Autodesk Inventor part; units mm, degrees
ref_plane "Work Plane1" through (0, 0, 10) normal (0, 0, 1) x (1, 0, 0)
ref_plane "YZ Plane" through (0, 0, 0) normal (1, 0, 0) x (0, 1, 0)
ref_plane "XZ Plane" through (0, 0, 0) normal (0, 1, 0) x (-1, 0, 0)
ref_plane "Work Plane1" through (0, 0, 10) normal (0, 0, 1) x (1, 0, 0)
sketch "Sketch2" plane through (0, 0, 10) normal (0, 0, 1) x (1, 0, 0)
  line L0 (0, 0) -> (30, 0)
  line L1 (30, 0) -> (30, 3)
  line L2 (30, 3) -> (0, 3)
  line L3 (0, 3) -> (0, 0)
  line L4 (30, 13) -> (0, 13)
  dimension "d11" = 30
  dimension "d12" = 3
  dimension "d13" = 10
revolve "Revolution1" add sketch "Sketch2" angle 360 about axis through (30, 13, 10) along (-1, 0, 0)
sketch "Sketch3" plane through (0, 0, 10) normal (0, 0, 1) x (1, 0, 0)
  line L0 (18.6699, 0) -> (35.6699, 0)
  line L1 (35.6699, 0) -> (35.6699, 5)
  line L2 (35.6699, 5) -> (18.6699, 5)
  line L3 (18.6699, 5) -> (28, 2.5)
  line L4 (28, 2.5) -> (18.6699, 0)
  line L5 (0, 26) -> (0, 0)
  line L6 (-3.0148, 0) -> (-5.3111, 0)
  dimension "d17" = 17
  dimension "d19" = 15
  dimension "d20" = 15
  dimension "d21" = 2.5
  dimension "d23" = 28
  dimension "d24" = 5
  dimension "d25" = 5.3111
  dimension "d26" = 7.6699
extrude "Extrusion2" cut sketch "Sketch3" along normal mid plane 13
equation "\"d20\" = d19"
properties part number "Whistle 1.3"
Build history of the part. All positions in model axes, mm. A direction names the side the tool comes from. Round coordinates to 2 decimals unless told otherwise and drop trailing zeros. Loops run counter-clockwise (first coordinate to the right, second up) from the corner with the lowest first, then second, coordinate; pieces in that order, holes last. Notation, with made-up numbers: (9.5, 83.5) -> (67.5, 83.5) arc R21 ccw to (67.5, 102.5) -> close; hole circle Ø4 at (81.25, 16). An arc over 180 degrees is marked (long way). Use CSV: the item, a comma, the result in double quotes. Start each with the question number.
Q1. Mould opens along Y. For faces 4 (the face through (30, 23, 12)), 5 (the face through (15.21, 25.987, 9.428)), 6 (the face through (26.38, 2.934, 9.909)), 7 (the face through (15, 23, 10)) say: +Y half, -Y half, draft (parallel to the pull), parting line (faces both ways), or undercut.
Q2. Flat gauge pins, fed straight in: pin 1 Ø2 at (x, z) = (13, 0) entering from -Y; pin 2 Ø5 at (x, z) = (21.5, 4.5) entering from -Y; pin 3 Ø3.5 at (x, y) = (23.5, 3.5) entering from +Z. Where does each tip first touch, or does it go through?
Q3. Which spindle directions (+Z, -Z, +X, -X, +Y, -Y) get a long thin tool onto all of the face, cutting with end or side? Do faces 1 (the face through (27, 4, 16.5)), 2 (the face through (24.437, 1.545, 9.909)), 3 (the face through (0, 6, 2)). Say none if no direction does.
Q4. Saw through at C-C on x = 19.5. Give the cut face in (y, z), and give its area (3 significant figures).
Q5. Saw through at B-B on z = 5. Give the cut face in (x, y), and give its area (3 significant figures).
Q6. Drill centre lines: L1, parallel to Y at x = 9, z = 10; L2, parallel to Z at x = 6.5, y = 13; L3, parallel to Y at x = 27.5, z = 15. Where is each one in solid material? Low to high.
Q7. Saw through at D-D on y = 8.25. Give the cut face in (x, z).
Q8. Saw through at A-A on y = 13. Give the cut face in (x, z).
Solutions:
1,face 4,"draft"
1,face 5,"parting line"
1,face 6,"undercut"
1,face 7,"undercut"
2,pin 1,"stops at y = 3.62"
2,pin 2,"stops at y = 0.43"
2,pin 3,"stops at z = 20.44"
3,face 1,"+X"
3,face 2,"+X, -Y"
3,face 3,"+Z, -Z, -X, +Y, -Y"
4,outline,"(0.22, 7.61) arc R13 ccw (long way) to (0.22, 12.39) -> close; hole (4.78, 3.5) -> (5, 3.5) -> (5, 4) arc R10 ccw (long way) to (5, 16) -> (5, 16.5) -> (4.78, 16.5) -> (4.78, 15.69) arc R10 ccw to (4.78, 4.31) -> close"
4,area,"216 mm^2"
5,outline,"(0, 1) -> (22.4, 1) -> (28, 2.5) -> (21.13, 4.34) -> (0, 4.34) -> close; (0, 21.66) -> (30, 21.66) -> (30, 25) -> (0, 25) -> close"
5,area,"183 mm^2"
6,L1,"y = 0 to 3, 23 to 26"
6,L2,"z = -3 to 0, 20 to 23"
6,L3,"y = 2.37 to 2.63, 21.66 to 25"
7,outline,"(0, -2.1) -> (30, -2.1) -> (30, 1.2) -> (0, 1.2) -> close; (0, 18.8) -> (30, 18.8) -> (30, 22.1) -> (0, 22.1) -> close"
8,outline,"(0, -3) -> (30, -3) -> (30, 0) -> (0, 0) -> close; (0, 20) -> (30, 20) -> (30, 23) -> (0, 23) -> close"
